Verification items for the finished model (mm, model axes). Round coordinates to 2 decimals unless told otherwise and drop trailing zeros. Order: outer loops, then holes, each group sorted by start corner. A loop starts at its lowest first (then second) coordinate and runs counter-clockwise, first axis right, second up. Notation, with made-up numbers: M 19,20.25 L 49,20.25 A13 cw 49,25.25 Z; hole C -4.5,-30 d8. An arc over 180 degrees is marked long. Use one line per item in the form item = value. Start each with the question number.
Item 1: Cross-section at B-B on z = 0. Enter the section's corners in (x, y) (3 decimals), then the cut area to 3 significant figures.
Item 2: Cross-section at C-C on z = -44.45. Enter the section's corners in (x, y) (3 decimals), then the cut area to 3 significant figures.
Item 3: Thickness scan on probe 1 along Y at (x, z) = (-1, -44.45) (3 decimals); probe 2 along Y at (x, z) = (1.75, 0) (3 decimals); probe 3 along Z at (x, y) = (-1, -35.5) (3 decimals). Record the ranges inside material, lowest first. Write a range as [from, to].
Item 4: Go/stop test with a flat-tipped pin: pin 1 Ø17 at (y, z) = (-30.36, 0) entering from +X. Record where the tip stops, or that it passes through.
Item 5: Cross-section at A-A on y = 44.45. Enter the section's corners in (x, z) (3 decimals).
Item 6: Cross-section at D-D on x = 1. Count the separate pieces of the cut face and the enclosed holes in it, then the cut area to 3 significant figures.
from build123d import *

# Parameters (mm, degrees)
SKETCH1_W           = 107.95
SKETCH1_H           = 107.95
SKETCH1_R           = 3.175
SKETCH1_R_2         = 14.2875
BOSS_EXTRUDE1_DEPTH = 3.175


with BuildPart() as part:
    # Sketch1 → Boss-Extrude1 (new, symmetric)
    with BuildSketch(Plane(origin=(0, 0, 0), x_dir=(0, 0, -1), z_dir=(1, 0, 0))):
        Rectangle(SKETCH1_W, SKETCH1_H)
        with Locations((-44.45, 44.45)):
            Circle(SKETCH1_R, mode=Mode.SUBTRACT)
        with Locations((-44.45, -19.05)):
            Circle(SKETCH1_R, mode=Mode.SUBTRACT)
        with Locations((-44.45, -44.45)):
            Circle(SKETCH1_R, mode=Mode.SUBTRACT)
        with Locations((44.45, -44.45)):
            Circle(SKETCH1_R, mode=Mode.SUBTRACT)
        with Locations((44.45, -19.05)):
            Circle(SKETCH1_R, mode=Mode.SUBTRACT)
        with Locations((44.45, 44.45)):
            Circle(SKETCH1_R, mode=Mode.SUBTRACT)
        with Locations((0, -30.357466082)):
            Circle(SKETCH1_R_2, mode=Mode.SUBTRACT)
    extrude(amount=BOSS_EXTRUDE1_DEPTH, both=True)


solid = part.part
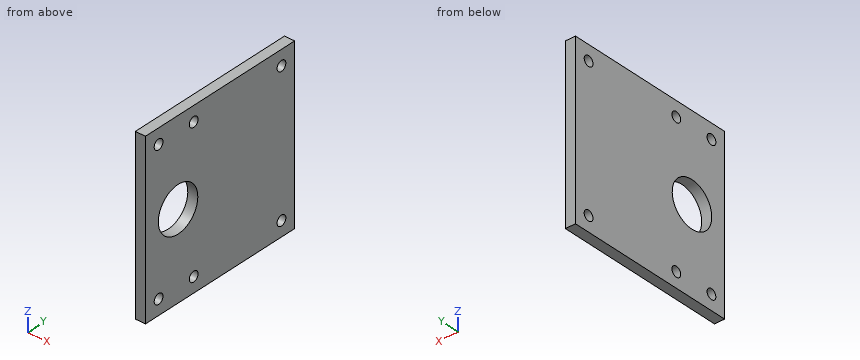
Output values:
q1.outline = M -3.175,-53.975 L 3.175,-53.975 L 3.175,-44.645 L -3.175,-44.645 Z; M -3.175,-16.07 L 3.175,-16.07 L 3.175,53.975 L -3.175,53.975 Z
q1.area = 504 mm2
q2.outline = M -3.175,-53.975 L 3.175,-53.975 L 3.175,-47.625 L -3.175,-47.625 Z; M -3.175,-41.275 L 3.175,-41.275 L 3.175,-22.225 L -3.175,-22.225 Z; M -3.175,-15.875 L 3.175,-15.875 L 3.175,41.275 L -3.175,41.275 Z; M -3.175,47.625 L 3.175,47.625 L 3.175,53.975 L -3.175,53.975 Z
q2.area = 565 mm2
q3.probe_1 = [-53.975, -47.625], [-41.275, -22.225], [-15.875, 41.275], [47.625, 53.975]
q3.probe_2 = [-53.975, -44.645], [-16.07, 53.975]
q3.probe_3 = [-53.975, -13.33], [13.33, 53.975]
q4.pin_1 = through
q5.outline = M -3.175,-53.975 L 3.175,-53.975 L 3.175,-47.625 L -3.175,-47.625 Z; M -3.175,-41.275 L 3.175,-41.275 L 3.175,41.275 L -3.175,41.275 Z; M -3.175,47.625 L 3.175,47.625 L 3.175,53.975 L -3.175,53.975 Z
q6.separate_pieces = 1
q6.enclosed_holes = 7
q6.area = 10,800 mm2
